from build123d import *

# Parameters (mm, degrees)
F0_W      = 60
F0_H      = 230
F1_DEPTH  = 10
F2_W      = 60
F2_H      = 10
F3_DEPTH  = 30
F4_R      = 3.25
F5_DEPTH  = 10.001
F6_W      = 60
F6_H      = 10
F7_DEPTH  = 80
F8_W      = 60
F8_H      = 10
F9_DEPTH  = 50
F10_R     = 3.25
F11_DEPTH = 10.001
F13_DEPTH = 230.001
F15_DEPTH = 5
F16_SIZE  = 2


with BuildPart() as f1:
    # F0 (on Front) → F1 (new body)
    with BuildSketch(Plane.XZ):
        Rectangle(F0_W, F0_H)
    extrude(amount=F1_DEPTH)

    # F2 (on face) → F3 (join)
    with BuildSketch(Plane(origin=(0, 0, 0), x_dir=(-1, 0, 0), z_dir=(0, 1, 0))):
        with Locations((0, -110)):
            Rectangle(F2_W, F2_H)
    extrude(amount=F3_DEPTH)

    # F4 (on face) → F5 (cut, through all)
    with BuildSketch(Plane.XY.offset(-105)):
        with Locations((20, 15)):
            Circle(F4_R)
        with Locations((-20, 15)):
            Circle(F4_R)
    extrude(amount=-F5_DEPTH, mode=Mode.SUBTRACT)

    # F6 (on face) → F7 (join)
    with BuildSketch(Plane.XZ.offset(10)):
        with Locations((0, 110)):
            Rectangle(F6_W, F6_H)
    extrude(amount=F7_DEPTH)

    # F8 (on face) → F9 (join)
    with BuildSketch(Plane.XZ.offset(10)):
        with Locations((0, -110)):
            Rectangle(F8_W, F8_H)
    extrude(amount=F9_DEPTH)

    # F10 (on face) → F11 (cut, through all)
    with BuildSketch(Plane.XY.offset(-105)):
        with Locations((20, -45)):
            Circle(F10_R)
        with Locations((-20, -45)):
            Circle(F10_R)
    extrude(amount=-F11_DEPTH, mode=Mode.SUBTRACT)

    # F12 (on face) → F13 (cut, through all)
    with BuildSketch(Plane.XY.offset(115)):
        with BuildLine():
            Line((3.4, -90), (3.4, -80))
            ThreePointArc((3.4, -80), (0, -76.6), (-3.4, -80))
            Line((-3.4, -80), (-3.4, -90))
            Line((-3.4, -90), (0, -90))
            Line((0, -90), (3.4, -90))
        make_face()
    extrude(amount=-F13_DEPTH, mode=Mode.SUBTRACT)

    # F14 (on face) → F15 (cut)
    with BuildSketch(Plane.XY.offset(115)):
        with BuildLine():
            Line((5.8, -90), (5.8, -80))
            ThreePointArc((5.8, -80), (0, -74.2), (-5.8, -80))
            Line((-5.8, -80), (-5.8, -90))
            Line((-5.8, -90), (5.8, -90))
        make_face()
    extrude(amount=-F15_DEPTH, mode=Mode.SUBTRACT)

    # F16
    f16_edges = [f1.edges().sort_by_distance(p)[0] for p in [
        (3.4, -90, 107.5),
        (-3.4, -90, 107.5),
        (5.8, -90, 112.5),
        (-5.8, -90, 112.5),
    ]]
    chamfer(f16_edges, length=F16_SIZE)


solid = f1.part
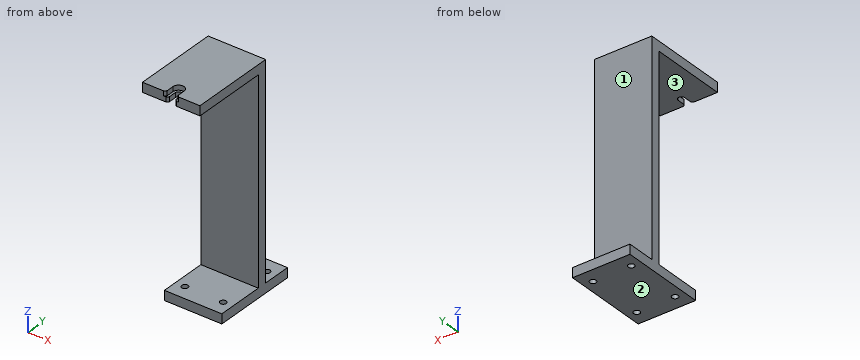
Could you check a few things on this model? Use its own coordinates, in mm. Face numbers are marked on the shaded views. A direction names the side the tool comes from. Give positions to 0.01 mm unless a question says otherwise; leave off trailing zeros. Write each loop counter-clockwise with the first axis right and the second up, starting at its lowest first coordinate (ties: lowest second). Pieces come first, ordered by that corner, then holes. Notation, with made-up numbers: (84, 6.25) -> (142, 6.25) arc R33 cw to (142, 44.25) -> close; hole circle Ø9 at (-23.5, -9.75). An arc over 180 degrees is marked (long way). Answer as a JSON object with one key per item and string values.
Q1. Please list where these lines run through material, in increasing order: L1, parallel to Y at x = 20, z = -111; L2, parallel to Z at x = -18, y = -29; L3, parallel to Y at x = -11, z = 104.
Taken from the geometry:
{"L1": "y = -60 to -48.25, -41.75 to 11.75, 18.25 to 30", "L2": "z = -115 to -105, 105 to 115", "L3": "y = -10 to 0"}
Q2. Suppose I cut it at C-C on x = -10.5. Write out the boundary of the cut face in (y, z).
Taken from the geometry:
{"outline": "(-90, 105) -> (-10, 105) -> (-10, -105) -> (-60, -105) -> (-60, -115) -> (30, -115) -> (30, -105) -> (0, -105) -> (0, 115) -> (-90, 115) -> close"}
Q3. Suppose I cut it at B-B on y = -45. Write out the boundary of the cut face in (x, z), then the cut area to 3 significant figures.
Taken from the geometry:
{"outline": "(-30, -115) -> (-23.25, -115) -> (-23.25, -105) -> (-30, -105) -> close; (-30, 105) -> (30, 105) -> (30, 115) -> (-30, 115) -> close; (-16.75, -115) -> (16.75, -115) -> (16.75, -105) -> (-16.75, -105) -> close; (23.25, -115) -> (30, -115) -> (30, -105) -> (23.25, -105) -> close", "area": "1,070 mm²"}
Q4. Which directions (+Z, -Z, +X, -X, +Y, -Y) give clear straight access to the entire face, cutting with the end or side of a thin tool? Please do the marked faces 1, 2 and 3.
Taken from the geometry:
{"face 1": "+Z, +X, -X, +Y", "face 2": "-Z, +X, -X, +Y, -Y", "face 3": "+X, -X, -Y"}
Q5. Will these pins go through, and if not, where does the flat tip stop? pin 1 Ø2 at (x, z) = (6, -68.5) entering from +Y; pin 2 Ø5 at (x, z) = (-1.5, 4.5) entering from -Y; pin 3 Ø3 at (x, z) = (2, -112) entering from -Y.
Taken from the geometry:
{"pin 1": "stops at y = 0", "pin 2": "stops at y = -10", "pin 3": "stops at y = -60"}
Q6. Suppose I cut it at A-A on x = -20. Write out the boundary of the cut face in (y, z), then the cut area to 3 significant figures.
Taken from the geometry:
{"outline": "(-90, 105) -> (-10, 105) -> (-10, -105) -> (-41.75, -105) -> (-41.75, -115) -> (11.75, -115) -> (11.75, -105) -> (0, -105) -> (0, 115) -> (-90, 115) -> close; (-60, -115) -> (-48.25, -115) -> (-48.25, -105) -> (-60, -105) -> close; (18.25, -115) -> (30, -115) -> (30, -105) -> (18.25, -105) -> close", "area": "3,770 mm²"}
Q7. Suppose I cut it at D-D on z = 50.5. Write out the boundary of the cut face in (x, y), then the cut area to 3 significant figures.
Taken from the geometry:
{"outline": "(-30, -10) -> (30, -10) -> (30, 0) -> (-30, 0) -> close", "area": "600 mm²"}
